from build123d import *

# Parameters (mm, degrees)
SKETCH1_R                = 25.4
SKETCH1_R_2              = 10
BOSS_EXTRUDE1_DEPTH      = 5
SKETCH1_R_3              = 13.95
SKETCH1_R_4              = 8
BOSS_EXTRUDE1_2_DEPTH    = 5
BOSS_EXTRUDE2_DEPTH      = 4
BOSS_EXTRUDE3_DEPTH      = 3
SKETCH3_R                = 20
SKETCH3_R_2              = 10
BOSS_EXTRUDE4_DEPTH      = 15
BOSS_EXTRUDE4_DEPTH_BACK = 25
CUT_EXTRUDE1_DEPTH       = 27.5
SCALE2_SCALE             = 0.1


with BuildPart() as part:
    # Sketch1 → Boss-Extrude1 (new body, symmetric)
    with BuildSketch(Plane.XY):
        with Locations((1.863247881, -32.575734897)):
            Circle(SKETCH1_R)
        with Locations((1.863247881, -32.575734897)):
            Circle(SKETCH1_R_2, mode=Mode.SUBTRACT)
    extrude(amount=BOSS_EXTRUDE1_DEPTH, both=True)



with BuildPart() as body_2:
    # Sketch1 → Boss-Extrude1 2 (new body, symmetric)
    with BuildSketch(Plane.XY):
        with Locations((1.863247881, 104.324265103)):
            Circle(SKETCH1_R_3)
        with Locations((1.863247881, 104.324265103)):
            Circle(SKETCH1_R_4, mode=Mode.SUBTRACT)
    extrude(amount=BOSS_EXTRUDE1_2_DEPTH, both=True)


with BuildPart() as part_1:
    add(part.part)

    add(body_2.part)  # Boss-Extrude2 merges body 2
    # Sketch1_3 → Boss-Extrude2 (add, symmetric)
    with BuildSketch(Plane.XY):
        with BuildLine():
            ThreePointArc((9.363247881, 92.561931151), (1.863247881, 90.374265103), (-5.636752119, 92.561931151))
            Line((-5.636752119, 92.561931151), (-14.636752119, -13.264857133))
            ThreePointArc((-14.636752119, -13.264857133), (1.863247881, -7.175734897), (18.363247881, -13.264857133))
            Line((18.363247881, -13.264857133), (9.363247881, 92.561931151))
        make_face()
        with BuildLine():
            ThreePointArc((-3.136752119, 74.324265103), (1.863247881, 79.324265103), (6.863247881, 74.324265103))
            Line((6.863247881, 74.324265103), (6.863247881, 7.424265103))
            ThreePointArc((6.863247881, 7.424265103), (1.863247881, 2.424265103), (-3.136752119, 7.424265103))
            Line((-3.136752119, 7.424265103), (-3.136752119, 74.324265103))
        make_face(mode=Mode.SUBTRACT)
    extrude(amount=BOSS_EXTRUDE2_DEPTH, both=True)

    # Sketch1_4 → Boss-Extrude3 (add, symmetric)
    with BuildSketch(Plane.XY):
        with BuildLine():
            Line((-3.136752119, 74.324265103), (-3.136752119, 7.424265103))
            ThreePointArc((-3.136752119, 7.424265103), (1.863247881, 2.424265103), (6.863247881, 7.424265103))
            Line((6.863247881, 7.424265103), (6.863247881, 74.324265103))
            ThreePointArc((6.863247881, 74.324265103), (1.863247881, 79.324265103), (-3.136752119, 74.324265103))
        make_face()
    extrude(amount=BOSS_EXTRUDE3_DEPTH, both=True)

    # Sketch3 → Boss-Extrude4 (add, two sides)
    with BuildSketch(Plane.XY.offset(5)) as boss_extrude4_sk:
        with Locations((1.863247881, -32.575734897)):
            Circle(SKETCH3_R)
        with Locations((1.863247881, -32.575734897)):
            Circle(SKETCH3_R_2, mode=Mode.SUBTRACT)
    extrude(amount=BOSS_EXTRUDE4_DEPTH)
    extrude(boss_extrude4_sk.sketch, amount=-BOSS_EXTRUDE4_DEPTH_BACK)

    # Sketch4 → Cut-Extrude1 (cut, symmetric)
    with BuildSketch(Plane.XY):
        with BuildLine():
            Line((-5.636752119, 92.561931151), (-25.096940363, -6.510465862))
            ThreePointArc((-25.096940363, -6.510465862), (1.863247881, -70.075734897), (28.823436125, -6.510465862))
            Line((28.823436125, -6.510465862), (9.363247881, 92.561931151))
            Line((9.363247881, 92.561931151), (17.863247881, -25.487011458))
            ThreePointArc((17.863247881, -25.487011458), (1.863247881, -50.075734897), (-14.136752119, -25.487011458))
            Line((-14.136752119, -25.487011458), (-5.636752119, 92.561931151))
        make_face()
    extrude(amount=CUT_EXTRUDE1_DEPTH, both=True, mode=Mode.SUBTRACT)


with BuildPart() as part_2:
    # Scale2: scaled about (1.863247881, 1.50194237, 0)
    add(part_1.part.scale(SCALE2_SCALE).moved(Location((1.676923093, 1.351748133, 0))))


solid = part_2.part
The listing builds one solid part. Answer for the finished solid, in the listing's coordinates (mm). A direction names the side the tool comes from. Round coordinates to 2 decimals unless told otherwise and drop trailing zeros. Order: outer loops, then holes, each group sorted by start corner. A loop starts at its lowest first (then second) coordinate and runs counter-clockwise, first axis right, second up. Notation, with made-up numbers: (0, -16) -> (5, -16) arc R32 ccw to (5, 17) -> close; hole circle Ø9 at (74, -15.5). An arc over 180 degrees is marked (long way). One line per item, written item: value.
Item 1: Find section B-B, the plane y = 12. Give the vertices of the cut face in (x, z), then the cut area to 3 significant figures.
Taken from the geometry:
outline: (0.49, -0.5) -> (1.09, -0.5) -> (1.09, 0.5) -> (0.49, 0.5) -> close; (2.63, -0.5) -> (3.24, -0.5) -> (3.24, 0.5) -> (2.63, 0.5) -> close
area: 1.22 mm2
Item 2: Given P1, Ø1.1, axis at x = 2, y = 7, coming from the -Z side; P2, Ø1.5, axis at x = 2.5, z = -1, coming from the +Y side; P3, Ø2, axis at x = 1.86, y = 11.78, coming from the +Z side, each flat-ended and moving along its own axis, determine where each tip first touches the part or whether it passes through.
Taken from the geometry:
P1: stops at z = -0.4
P2: stops at y = 13.18
P3: stops at z = 0.5
Item 3: For a pull along X with two mould halves and no side action, classify faces 1 (the flat face through (1.8, 0.3, -0.5)), 2 (the cylindrical face through (1.888, 0.094, -1.24)), 3 (the flat face through (2, 5, 0.3)) as released by +X, released by -X, zero draft, split by the parting line, or undercut.
Taken from the geometry:
face 1: zero draft
face 2: split by the parting line
face 3: undercut
Item 4: Find section C-C, the plane x = 2.15. State how many separate pieces and enclosed holes the cut face has, then the cut area to 3 significant figures.
Taken from the geometry:
separate pieces: 3
enclosed holes: 0
area: 15.3 mm2
Item 5: Find section A-A, the plane x = 3.1. Give the vertices of the cut face in (y, z), then the cut area to 3 significant figures.
Taken from the geometry:
outline: (-3.14, -2) -> (-0.33, -2) -> (-0.33, -0.5) -> (0.31, -0.5) -> (0.31, -0.4) -> (3.85, -0.4) -> (3.85, 0.4) -> (0.31, 0.4) -> (0.31, 0.5) -> (-0.33, 0.5) -> (-0.33, 2) -> (-3.14, 2) -> close; (11.14, -0.5) -> (12.43, -0.5) -> (12.43, 0.5) -> (11.14, 0.5) -> close
area: 16.0 mm2
Item 6: For faces 4 (the flat face through (1.8, 0.3, 0.5)), 5 (the flat face through (2, 5, -0.3)), 6 (the flat face through (3, 12, -0.5)), 7 (the flat face through (0.623, 3.804, -0.139)), determine the directions among +Z, -Z, +X, -X, +Y, -Y from which every point of the face is accessible in a straight line to the end or side of a thin tool.
Taken from the geometry:
face 4: +Z, +Y
face 5: -Z
face 6: -Z, +X, -X, +Y
face 7: +Z, -Z, -X
Item 7: Straight lines are drawn through the part: L1, parallel to Y at x = 2.6, z = 1.8; L2, parallel to Y at x = 1.35, z = 1.1; L3, parallel to X at y = -1, z = -0.95. For each, find the intervals that lie inside material, in ascending order.
Taken from the geometry:
L1: y = -3.49 to -2.58, -1.23 to -0.05
L2: y = -3.58 to -2.76, -1.05 to 0.03
L3: x = 0.28 to 1.44, 2.29 to 3.45
Item 8: Find section D-D, the plane z = -0.85. Give the vertices of the cut face in (x, y).
Taken from the geometry:
outline: (0.26, -1.2) arc R1.75 ccw (long way) to (3.46, -1.2) -> (3.42, -0.66) arc R2 ccw to (0.3, -0.66) -> close; hole circle Ø2 at (1.86, -1.91)
